Design review of the part built by this model. Coordinates are the model's own, in mm. A direction names the side the tool comes from. Coordinates: 2 decimals unless noted, no trailing zeros. Order: outer loops, then holes, each group sorted by start corner. A loop starts at its lowest first (then second) coordinate and runs counter-clockwise, first axis right, second up. Notation, with made-up numbers: M 57,-15 L 89,-15 A8 cw 89,-5 Z; hole C -40,20 d3. An arc over 180 degrees is marked long. Answer in a Markdown table with one row per item.
from build123d import *

# Parameters (mm, degrees)
BOSS_EXTRUDE1_DEPTH = 15
SKETCH2_W           = 11
SKETCH2_H           = 11
CUT_EXTRUDE1_DEPTH  = 80.765427423
CUT_EXTRUDE2_DEPTH  = 136.155378328
SKETCH4_R           = 1.6
CUT_EXTRUDE3_DEPTH  = 132.425469972


with BuildPart() as part:
    # Sketch1 → Boss-Extrude1 (new body)
    with BuildSketch(Plane(origin=(0, 0, 0), x_dir=(1, 0, 0), z_dir=(0, 1, 0))):
        Polygon((130, 19.30425231), (126.117714323, 33.793139704), (54.073263901, 14.488887394), (57.955549577, 0), align=None)
    extrude(amount=BOSS_EXTRUDE1_DEPTH)

    # Sketch2 → Cut-Extrude1 (cut, through all)
    with BuildSketch(Plane(origin=(54.073263901, 0, -14.488887394), x_dir=(-0.2588190451025183, 0, -0.965925826289069), z_dir=(0.965925826289069, 0, -0.2588190451025183))):
        with Locations((-7.5, 7.5)):
            Rectangle(SKETCH2_W, SKETCH2_H)
    extrude(amount=CUT_EXTRUDE1_DEPTH, mode=Mode.SUBTRACT)

    # Sketch3 → Cut-Extrude2 (cut, through all)
    with BuildSketch(Plane(origin=(0, 15, 0), x_dir=(1, 0, 0), z_dir=(0, 1, 0))):
        Polygon((126.117714323, 33.793139704), (126.117714323, 18.263996998), (130, 19.30425231), align=None)
        Polygon((54.073263901, 14.488887394), (57.955549577, 15.529142706), (57.955549577, 0), align=None)
    extrude(amount=-CUT_EXTRUDE2_DEPTH, mode=Mode.SUBTRACT)

    # Sketch4 → Cut-Extrude3 (cut, through all)
    with BuildSketch(Plane.XZ):
        with Locations(Location((118.617714323, -24.018949408, 0), (0, 0, 270))):
            Circle(SKETCH4_R)
        with Locations(Location((65.455549577, -9.774190296, 0), (0, 0, 270))):
            Circle(SKETCH4_R)
    extrude(amount=-CUT_EXTRUDE3_DEPTH, mode=Mode.SUBTRACT)


solid = part.part
(1) Draft analysis for pull direction Z (two halves, no side actions). For faces 1 (the flat face through (91.559, 7.395, -9.004)), 2 (the flat face through (92, 13, -17)), 3 (the flat face through (126.118, 14, -26)), 4 (the flat face through (92, 2, -17)), state which applies: pulls with the +Z half, pulls with the -Z half, needs draft (parallel to the pull), parting line crosses it, or undercut.
Return value:
| item | result |
|---|---|
| face 1 | pulls with the +Z half |
| face 2 | undercut |
| face 3 | needs draft |
| face 4 | undercut |
(2) For faces 5 (the flat face through (91.559, 7.423, -22.463)), 6 (the flat face through (92, 0, -17)), list the 3-axis set-ups (+Z, -Z, +X, -X, +Y, -Y) from which the entire face can be reached by the end or side of a thin tool; tool diameter is ignored.
Return value:
| item | result |
|---|---|
| face 5 | none |
| face 6 | +Z, -Z, +X, -X, -Y |
(3) For line 1 along Y through (x, z) = (104.5, -22.5); line 2 along Z through (x, y) = (108, 7); line 3 along Z through (x, y) = (89.5, 5.75), list the stretches that pass through material, from the lowest coordinate up. Write a range as from..to.
Return value:
| item | result |
|---|---|
| line 1 | y = 0..2, 13..15 |
| line 2 | z = -28.94..-26.87, -15.48..-13.41 |
| line 3 | z = -23.98..-21.91, -10.52..-8.45 |
(4) Add section D-D, the plane z = -17.5. Give the boundary of the cut face in (x, y).
Return value:
| item | result |
|---|---|
| outline | M 65.31,0 L 123.27,0 L 123.27,15 L 65.31,15 Z; hole M 73.04,2 L 115.54,2 L 115.54,13 L 73.04,13 Z |
(5) Add section C-C, the plane x = 90. Give the boundary of the cut face in (y, z).
Return value:
| item | result |
|---|---|
| outline | M 0,-24.12 L 15,-24.12 L 15,-8.59 L 0,-8.59 Z; hole M 2,-22.04 L 13,-22.04 L 13,-10.66 L 2,-10.66 Z |
(6) Add section A-A, the plane y = 10.75. Give the boundary of the cut face in (x, z).
Return value:
| item | result |
|---|---|
| outline | M 57.96,-15.53 L 126.12,-33.79 L 126.12,-31.72 L 57.96,-13.46 Z; M 57.96,-2.07 L 126.12,-20.33 L 126.12,-18.26 L 57.96,0 Z |
(7) Insertion check: pin 1 Ø2.5 at (x, z) = (118.62, -24.02) entering from -Y; pin 2 Ø8 at (x, y) = (101, 2) entering from -Z; pin 3 Ø1.5 at (x, y) = (98, 11.5) entering from -Z. Each pin has a flat end and moves straight along its axis. Give the tip position at first contact, or say it passes through.
Return value:
| item | result |
|---|---|
| pin 1 | passes through |
| pin 2 | stops at z = -28.13 |
| pin 3 | stops at z = -26.46 |
(8) Add section B-B, the plane z = -9. Give the boundary of the cut face in (x, y).
Return value:
| item | result |
|---|---|
| outline | M 57.96,0 L 64.06,0 L 64.06,2 L 57.96,2 Z; M 57.96,13 L 64.06,13 L 64.06,15 L 57.96,15 Z; M 66.86,0 L 91.54,0 L 91.54,15 L 66.86,15 L 66.86,13 L 83.82,13 L 83.82,2 L 66.86,2 Z |
